from build123d import *

# Parameters (mm, degrees)
F1_DEPTH = 4


# Not quite as in the source:
# - ends of sketch curves that miss each other by under 0.0002 mm in the source are joined


with BuildPart() as f1:
    # F0 (on Front) → F1 (new body)
    with BuildSketch(Plane.XZ):
        with BuildLine():
            Line((0, -60.8297549188), (0, -73.8967955112))
            Line((0, -73.8967955112), (87.1100496289, -74.2867405805))
            Line((87.1100496289, -74.2867405805), (101.0242826289, -67.1413325805))
            Line((101.0242826289, -67.1413325805), (105.9525546289, -57.2604655805))
            Line((105.9525546289, -57.2604655805), (106.3312226289, -19.1988875805))
            Line((106.3312226289, -19.1988875805), (108.1210446289, -19.0793755805))
            Line((108.1210446289, -19.0793755805), (108.5219496289, 39.4283344195))
            Line((108.5219496289, 39.4283344195), (106.4708796289, 39.5943924195))
            Line((106.4708796289, 39.5943924195), (106.4000046289, 73.4808784195))
            Line((106.4000046289, 73.4808784195), (92.8644466289, 73.6712574195))
            Line((92.8644466289, 73.6712574195), (92.6761516289, 76.0280454195))
            Line((92.6761516289, 76.0280454195), (77.0874396289, 76.0523674195))
            Line((77.0874396289, 76.0523674195), (77.0408646289, 73.7421304195))
            Line((77.0408646289, 73.7421304195), (54.5193526289, 73.8595534195))
            Line((54.5193526289, 73.8595534195), (54.4241656289, 76.0746004195))
            Line((54.4241656289, 76.0746004195), (0, 76.1053934693))
            Line((0, 76.1053934693), (0, 58.2839623094))
            Line((0, 58.2839623094), (56.1452326289, 58.5077654195))
            Line((56.1452326289, 58.5077654195), (56.4530356289, -19.0793755805))
            Line((56.4530356289, -19.0793755805), (40.5120526289, -19.1745575805))
            add(Edge.make_bspline(
                [(40.5120526289, -19.1745575805), (36.9506296289, -19.7234595805), (31.0349826289, -20.1211625805), (28.1548906289, -29.4563295805)],
                knots=[0, 0, 0, 0, 1, 1, 1, 1], degree=3))
            add(Edge.make_bspline(
                [(28.1548906289, -29.4563295805), (27.3785236289, -34.8808025805), (27.2311746289, -40.4625355805), (25.0629916289, -45.5390525805)],
                knots=[0, 0, 0, 0, 1, 1, 1, 1], degree=3))
            add(Edge.make_bspline(
                [(25.0629916289, -45.5390525805), (22.5362476289, -50.0321895805), (19.6081916289, -53.5319905805), (15.1727896289, -56.0456005805)],
                knots=[0, 0, 0, 0, 1, 1, 1, 1], degree=3))
            add(Edge.make_bspline(
                [(15.1727896289, -56.0456005805), (10.4594036477, -58.820394717), (5.445743624, -60.1029114405), (0.1550796733, -60.8297549188)],
                knots=[0, 0, 0, 0, 0.9984504356, 0.9984504356, 0.9984504356, 0.9984504356], degree=3))
            Line((0.1550796733, -60.8297549188), (0, -60.8297549188))
        make_face()
        Polygon((22.4935926289, -66.8113025805), (22.6353336289, -62.1665075805), (36.8552756289, -62.0956475805), (36.9483786289, -66.8821775805), align=None, mode=Mode.SUBTRACT)
        with BuildLine():
            Line((36.5252426289, -40.4245775805), (37.0456556289, -30.1386355805))
            add(Edge.make_bspline(
                [(47.9388526289, -30.2581405805), (47.5903856289, -26.1010925805), (40.1854096289, -22.9941275805), (37.0456556289, -30.1386355805)],
                knots=[0, 0, 0, 0, 1, 1, 1, 1], degree=3))
            Line((47.9388526289, -30.2581405805), (47.9166236289, -40.4245775805))
            add(Edge.make_bspline(
                [(36.5252426289, -40.4245775805), (39.5748886289, -47.0515105805), (46.1937256289, -46.0800805805), (47.9166236289, -40.4245775805)],
                knots=[0, 0, 0, 0, 1, 1, 1, 1], degree=3))
        make_face(mode=Mode.SUBTRACT)
        Polygon((52.3508896289, -66.8578555805), (52.5391806289, -62.3061655805), (70.6729776289, -62.2595755805), (70.8147186289, -66.8091795805), align=None, mode=Mode.SUBTRACT)
        with BuildLine():
            add(Edge.make_bspline(
                [(91.8478096289, -27.5109605805), (96.8262026289, -30.2957185805), (99.8930176289, -35.4421625805), (99.8930176289, -41.0116775805)],
                knots=[0, 0, 0, 0, 1, 1, 1, 1], degree=3))
            add(Edge.make_bspline(
                [(99.8930176289, -41.0116775805), (99.8930176289, -46.5811925805), (96.8262026289, -51.7276365805), (91.8478096289, -54.5123945805)],
                knots=[0, 0, 0, 0, 1, 1, 1, 1], degree=3))
            add(Edge.make_bspline(
                [(91.8478096289, -54.5123945805), (86.8694176289, -57.2971515805), (80.7357866289, -57.2971515805), (75.7573936289, -54.5123945805)],
                knots=[0, 0, 0, 0, 1, 1, 1, 1], degree=3))
            add(Edge.make_bspline(
                [(75.7573936289, -54.5123945805), (70.7790016289, -51.7276365805), (67.7121856289, -46.5811925805), (67.7121856289, -41.0116775805)],
                knots=[0, 0, 0, 0, 1, 1, 1, 1], degree=3))
            add(Edge.make_bspline(
                [(67.7121856289, -41.0116775805), (67.7121856289, -35.4421625805), (70.7790016289, -30.2957185805), (75.7573936289, -27.5109605805)],
                knots=[0, 0, 0, 0, 1, 1, 1, 1], degree=3))
            add(Edge.make_bspline(
                [(75.7573936289, -27.5109605805), (80.7357866289, -24.7262035805), (86.8694176289, -24.7262035805), (91.8478096289, -27.5109605805)],
                knots=[0, 0, 0, 0, 1, 1, 1, 1], degree=3))
        make_face(mode=Mode.SUBTRACT)
        with BuildLine():
            add(Edge.make_bspline(
                [(68.1673266289, 15.0146874195), (69.4436526289, 25.8273554195), (91.6549896289, 38.5868954195), (99.9389866289, 15.7162674195)],
                knots=[0, 0, 0, 0, 1, 1, 1, 1], degree=3))
            Line((99.9389866289, 15.7162674195), (100.1394466289, -4.5293975805))
            add(Edge.make_bspline(
                [(100.1394466289, -4.5293975805), (92.4962496289, -23.3266025805), (72.9593576289, -19.3084625805), (67.7664206289, -4.0282625805)],
                knots=[0, 0, 0, 0, 1, 1, 1, 1], degree=3))
            Line((67.7664206289, -4.0282625805), (68.1673266289, 15.0146874195))
        make_face(mode=Mode.SUBTRACT)
        with BuildLine():
            add(Edge.make_bspline(
                [(92.5110916289, 65.8933484195), (97.4657886289, 63.0685594195), (100.5180086289, 57.8481334195), (100.5180086289, 52.1985554195)],
                knots=[0, 0, 0, 0, 1, 1, 1, 1], degree=3))
            add(Edge.make_bspline(
                [(100.5180086289, 52.1985554195), (100.5180086289, 46.5489774195), (97.4657886289, 41.3285514195), (92.5110916289, 38.5037624195)],
                knots=[0, 0, 0, 0, 1, 1, 1, 1], degree=3))
            add(Edge.make_bspline(
                [(92.5110916289, 38.5037624195), (87.5563936289, 35.6789734195), (81.4519556289, 35.6789734195), (76.4972576289, 38.5037624195)],
                knots=[0, 0, 0, 0, 1, 1, 1, 1], degree=3))
            add(Edge.make_bspline(
                [(76.4972576289, 38.5037624195), (71.5425606289, 41.3285514195), (68.4903406289, 46.5489774195), (68.4903406289, 52.1985554195)],
                knots=[0, 0, 0, 0, 1, 1, 1, 1], degree=3))
            add(Edge.make_bspline(
                [(68.4903406289, 52.1985554195), (68.4903406289, 57.8481334195), (71.5425606289, 63.0685594195), (76.4972576289, 65.8933484195)],
                knots=[0, 0, 0, 0, 1, 1, 1, 1], degree=3))
            add(Edge.make_bspline(
                [(76.4972576289, 65.8933484195), (81.4519556289, 68.7181374195), (87.5563936289, 68.7181374195), (92.5110916289, 65.8933484195)],
                knots=[0, 0, 0, 0, 1, 1, 1, 1], degree=3))
        make_face(mode=Mode.SUBTRACT)
    extrude(amount=F1_DEPTH)

    # F2: F1 across plane


with BuildPart() as f1_1:
    add(f1.part)
    add(f1.part.mirror(Plane.YZ))


solid = f1_1.part
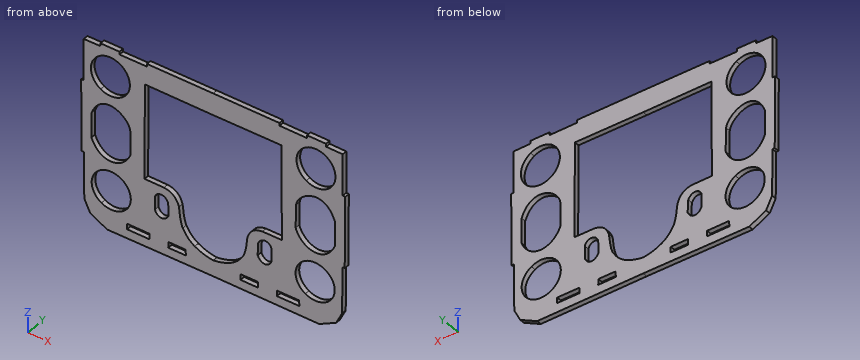
Model file for the job. Use its own axes, mm. Round coordinates to 2 decimals unless told otherwise and drop trailing zeros. Loops run counter-clockwise (first coordinate to the right, second up) from the corner with the lowest first, then second, coordinate; pieces in that order, holes last. Notation, with made-up numbers: M -14.75,70 L 34.25,70 A17 cw 34.25,82 Z; hole C 71,39 d2. An arc over 180 degrees is marked long. One line per question, with ' | ' between items.
1) Band-saw the part on B-B (z = 33). Give the cut face in (x, y).
Solved:
outline: M -108.48,-4 L -56.25,-4 L -56.25,0 L -108.48,0 Z; M 56.25,-4 L 108.48,-4 L 108.48,0 L 56.25,0 Z
2) Band-saw the part on D-D (y = -2.65). Give the number of separate pieces and of enclosed holes in the cut face, then the cut area to 3 significant figures.
Solved:
separate pieces: 1 | enclosed holes: 13 | area: 14,700 mm²
3) Band-saw the part on A-A (z = 12). Give the cut face in (x, y).
Solved:
outline: M -108.33,-4 L -99.98,-4 L -99.98,0 L -108.33,0 Z; M -68.1,-4 L -56.33,-4 L -56.33,0 L -68.1,0 Z; M 56.33,-4 L 68.1,-4 L 68.1,0 L 56.33,0 Z; M 99.98,-4 L 108.33,-4 L 108.33,0 L 99.98,0 Z
4) Band-saw the part on C-C (x = -62). Give the cut face in (y, z).
Solved:
outline: M -4,-74.17 L 0,-74.17 L 0,-66.83 L -4,-66.83 Z; M -4,-62.28 L 0,-62.28 L 0,73.82 L -4,73.82 Z
5) Flat gauge pins, fed straight in: pin 1 (1.5 mm diameter, centred on x = -44, y = -2, fed in from -Z); pin 2 (1 mm diameter, centred on x = -16.5, y = -3, fed in from -Z); pin 3 (1.5 mm diameter, centred on y = -2, z = -52.5, fed in from +X). Where does each tip first touch, or does it go through?
Solved:
pin 1: stops at z = -74.1 | pin 2: stops at z = -73.97 | pin 3: stops at x = 106.01
6) Drill centre lines: line 1 along Z through (x, y) = (-89, -2.05); line 2 along X through (y, z) = (-0.3, 8); line 3 along X through (y, z) = (-3.1, -14). Where is each one in solid material? Low to high.
Solved:
line 1: z = -73.32 to -55.77, -26.26 to -16.33, 27.91 to 37.02, 67.38 to 76.03 | line 2: x = -108.31 to -100.02, -68.02 to -56.35, 56.35 to 68.02, 100.02 to 108.31 | line 3: x = -108.16 to -93.32, -74.98 to -56.43, 56.43 to 74.98, 93.32 to 108.16
